from build123d import *

# Parameters (mm, degrees)
SALIENTE_EXTRUIR1_DEPTH = 15
CROQUIS2_W              = 159.5
CROQUIS2_H              = 106.5
SALIENTE_EXTRUIR2_DEPTH = 109.6
CORTAR_EXTRUIR1_DEPTH   = 5
CROQUIS4_R              = 4
CORTAR_EXTRUIR2_DEPTH   = 15
CROQUIS5_W              = 149.31449295
CROQUIS5_H              = 13.110540845
SALIENTE_EXTRUIR3_DEPTH = 11


with BuildPart() as part:
    # Croquis1 → Saliente-Extruir1 (new body)
    with BuildSketch(Plane.XY):
        with BuildLine():
            Line((-101.5, -70.5), (101.5, -70.5))
            ThreePointArc((101.5, -70.5), (108.571067812, -67.571067812), (111.5, -60.5))
            Line((111.5, -60.5), (111.5, 60.5))
            ThreePointArc((111.5, 60.5), (108.571067812, 67.571067812), (101.5, 70.5))
            Line((101.5, 70.5), (-101.5, 70.5))
            ThreePointArc((-101.5, 70.5), (-108.571067812, 67.571067812), (-111.5, 60.5))
            Line((-111.5, 60.5), (-111.5, -60.5))
            ThreePointArc((-111.5, -60.5), (-108.571067812, -67.571067812), (-101.5, -70.5))
        make_face()
    extrude(amount=SALIENTE_EXTRUIR1_DEPTH)

    # Croquis2 → Saliente-Extruir2 (add)
    with BuildSketch(Plane(origin=(0, 0, 0), x_dir=(-1, 0, 0), z_dir=(0, 0, -1))):
        Rectangle(CROQUIS2_W, CROQUIS2_H)
    extrude(amount=SALIENTE_EXTRUIR2_DEPTH)

    # Croquis3 → Cortar-Extruir1 (cut)
    with BuildSketch(Plane.XY.offset(15)):
        with BuildLine():
            Line((86.5, -55.5), (-86.5, -55.5))
            ThreePointArc((-86.5, -55.5), (-93.571067812, -52.571067812), (-96.5, -45.5))
            Line((-96.5, -45.5), (-96.5, 45.5))
            ThreePointArc((-96.5, 45.5), (-93.571067812, 52.571067812), (-86.5, 55.5))
            Line((-86.5, 55.5), (86.5, 55.5))
            ThreePointArc((86.5, 55.5), (93.571067812, 52.571067812), (96.5, 45.5))
            Line((96.5, 45.5), (96.5, -45.5))
            ThreePointArc((96.5, -45.5), (93.571067812, -52.571067812), (86.5, -55.5))
        make_face()
    extrude(amount=-CORTAR_EXTRUIR1_DEPTH, mode=Mode.SUBTRACT)

    # Croquis4 → Cortar-Extruir2 (cut)
    with BuildSketch(Plane.XY.offset(15)):
        with Locations((-103.5, 62.5)):
            Circle(CROQUIS4_R)
        with Locations((103.5, 62.5)):
            Circle(CROQUIS4_R)
        with Locations((103.5, -62.5)):
            Circle(CROQUIS4_R)
        with Locations((-103.5, -62.5)):
            Circle(CROQUIS4_R)
    extrude(amount=-CORTAR_EXTRUIR2_DEPTH, mode=Mode.SUBTRACT)

    # Croquis5 → Saliente-Extruir3 (add)
    with BuildSketch(Plane(origin=(0, 53.25, 0), x_dir=(1, 0, 0), z_dir=(0, 1, 0))):
        with Locations((0, 83.536078168)):
            Rectangle(CROQUIS5_W, CROQUIS5_H)
    extrude(amount=SALIENTE_EXTRUIR3_DEPTH)


solid = part.part
Can you work these out from the model? Positions are in its coordinate system, mm. A direction names the side the tool comes from. Coordinates: 2 decimals unless noted, no trailing zeros. Write each loop counter-clockwise with the first axis right and the second up, starting at its lowest first coordinate (ties: lowest second). Pieces come first, ordered by that corner, then holes. Notation, with made-up numbers: (-3, -1) - (48, -1) arc R19 cw to (48, 35) - close; hole circle Ø1 at (-18.75, 28.5). An arc over 180 degrees is marked (long way). Return JSON: item names as keys, results as strings. Group by question number.
Item 1: If we section it at C-C (z = -38): Write out the boundary of the cut face in (x, y).
Item 2: Please list where these lines run through material, in increasing order: probe 1 along Y at (x, z) = (-103, 3); probe 2 along Y at (x, z) = (103.5, 3.25); probe 3 along Y at (x, z) = (70.5, -8.5).
Item 3: Which directions (+Z, -Z, +X, -X, +Y, -Y) give clear straight access to the entire face, cutting with the end or side of a thin tool? Please do faces 1 (the face through (79.75, -1, -54)), 2 (the face through (-1, 59, -76.981)), 3 (the face through (93.65, -52.49, 12.54)), 4 (the face through (1, -53.25, -54)).
Item 4: If we section it at A-A (x = 6.5): Write out the boundary of the cut face in (y, z), then the cut area to 3 significant figures.
Item 5: I'm going to push flat-ended pins straight in: pin 1 Ø1 at (y, z) = (-34, -84.5) entering from -X; pin 2 Ø14.5 at (x, z) = (23.5, -80.5) entering from +Y; pin 3 Ø3 at (y, z) = (44.5, -36) entering from +X; pin 4 Ø10.5 at (x, y) = (103.5, 62.5) entering from +Z. Where does each tip first touch, or does it pass through?
Item 6: We'd pull the mould along Z, two halves only. Please class faces 5 (the face through (-96.5, -1, 13)), 6 (the face through (1, 1, 10)), 7 (the face through (1, 53.25, -54)): pulls with the +Z half, pulls with the -Z half, needs draft (parallel to the pull), parting line crosses it, or undercut.
Item 7: If we section it at B-B (y = 33): Write out the boundary of the cut face in (x, z).
Return value:
{
 "1": {"outline": "(-79.75, -53.25) - (79.75, -53.25) - (79.75, 53.25) - (-79.75, 53.25) - close"},
 "2": {"probe 1": "y = -70.39 to -66.47, -58.53 to 58.53, 66.47 to 70.39", "probe 2": "y = -70.3 to -66.5, -58.5 to 58.5, 66.5 to 70.3", "probe 3": "y = -53.25 to 53.25"},
 "3": {"face 1": "-Z, +X, +Y, -Y", "face 2": "+X, -X, +Y", "face 3": "+Z", "face 4": "-Z, +X, -X, -Y"},
 "4": {"outline": "(-70.5, 0) - (-53.25, 0) - (-53.25, -109.6) - (53.25, -109.6) - (53.25, -90.09) - (64.25, -90.09) - (64.25, -76.98) - (53.25, -76.98) - (53.25, 0) - (70.5, 0) - (70.5, 15) - (55.5, 15) - (55.5, 10) - (-55.5, 10) - (-55.5, 15) - (-70.5, 15) - close", "area": "13,400 mm^2"},
 "5": {"pin 1": "stops at x = -79.75", "pin 2": "stops at y = 64.25", "pin 3": "stops at x = 79.75", "pin 4": "stops at z = 15"},
 "6": {"face 5": "needs draft", "face 6": "pulls with the +Z half", "face 7": "undercut"},
 "7": {"outline": "(-111.5, 0) - (-79.75, 0) - (-79.75, -109.6) - (79.75, -109.6) - (79.75, 0) - (111.5, 0) - (111.5, 15) - (96.5, 15) - (96.5, 10) - (-96.5, 10) - (-96.5, 15) - (-111.5, 15) - close"}
}
